from build123d import *

# Parameters (mm, degrees)
SKETCH1_R           = 3
SKETCH1_R_2         = 5
BOSS_EXTRUDE1_DEPTH = 4
FILLET1_R           = 5
SKETCH2_R           = 5
BOSS_EXTRUDE2_DEPTH = 12
SKETCH4_R           = 2.401871641
CUT_EXTRUDE2_DEPTH  = 30
SKETCH6_R           = 2.15
CUT_EXTRUDE3_DEPTH  = 2.9


with BuildPart() as part:
    # Sketch1 → Boss-Extrude1 (new body)
    with BuildSketch(Plane(origin=(0, 0, 0), x_dir=(1, 0, 0), z_dir=(0, 1, 0))):
        Polygon((-5.790326763, 58.347363117), (-5.790326763, -9.85213545), (63.193084095, -9.85213545), align=None)
        with Locations(Location((2.52138652, 36.496379496, 0), (0, 0, 270))):
            Circle(SKETCH1_R, mode=Mode.SUBTRACT)
        with Locations(Location((34.519986489, 4.856379496, 0), (0, 0, 270))):
            Circle(SKETCH1_R_2, mode=Mode.SUBTRACT)
    extrude(amount=BOSS_EXTRUDE1_DEPTH)

    # Fillet1
    fillet1_edges = [part.edges().sort_by_distance(p)[0] for p in [
        (63.193084095, 2, 9.85213545),
        (-5.790326763, 2, -58.347363117),
    ]]
    fillet(fillet1_edges, radius=FILLET1_R)

    # Sketch2 → Boss-Extrude2 (add)
    # profile 1 of 5: a face of its own
    with BuildSketch(Plane(origin=(0, 4, 0), x_dir=(1, 0, 0), z_dir=(0, 1, 0))):
        with BuildLine():
            Line((42.017536623, -1.29645629), (54.539062539, -1.29645629))
            Line((54.539062539, -1.29645629), (41.338915092, 11.753687589))
            ThreePointArc((41.338915092, 11.753687589), (43.470054942, 8.593613888), (44.21898882, 4.856379496))
            ThreePointArc((44.21898882, 4.856379496), (43.65205642, 1.588973033), (42.017536623, -1.29645629))
        make_face()
    # profile 2 of 5: a face of its own
    with BuildSketch(Plane(origin=(0, 4, 0), x_dir=(1, 0, 0), z_dir=(0, 1, 0))):
        with BuildLine():
            ThreePointArc((51.023789334, -9.85213545), (55.648635051, -6.752346517), (54.539062539, -1.29645629))
            Line((54.539062539, -1.29645629), (42.017536623, -1.29645629))
            ThreePointArc((42.017536623, -1.29645629), (34.519986489, -4.842622834), (27.022436356, -1.29645629))
            Line((27.022436356, -1.29645629), (-5.790326763, -1.29645629))
            Line((-5.790326763, -1.29645629), (-5.790326763, -9.85213545))
            Line((-5.790326763, -9.85213545), (51.023789334, -9.85213545))
        make_face()
    # profile 3 of 5: a face of its own
    with BuildSketch(Plane(origin=(0, 4, 0), x_dir=(1, 0, 0), z_dir=(0, 1, 0))):
        with BuildLine():
            ThreePointArc((27.022436356, -1.29645629), (34.519986489, -4.842622834), (42.017536623, -1.29645629))
            Line((42.017536623, -1.29645629), (27.022436356, -1.29645629))
        make_face()
    # profile 4 of 5: a face of its own
    with BuildSketch(Plane(origin=(0, 4, 0), x_dir=(1, 0, 0), z_dir=(0, 1, 0))):
        with BuildLine():
            ThreePointArc((34.519986489, 14.555381827), (38.206016803, 13.827657373), (41.338915092, 11.753687589))
            Line((41.338915092, 11.753687589), (32.887372323, 20.109188887))
            Line((32.887372323, 20.109188887), (-5.790326763, 20.109188887))
            Line((-5.790326763, 20.109188887), (-5.790326763, 14.555381827))
            Line((-5.790326763, 14.555381827), (34.519986489, 14.555381827))
        make_face()
    # profile 5 of 5: a face of its own
    with BuildSketch(Plane(origin=(0, 4, 0), x_dir=(1, 0, 0), z_dir=(0, 1, 0))):
        with BuildLine():
            Line((27.022436356, -1.29645629), (42.017536623, -1.29645629))
            ThreePointArc((42.017536623, -1.29645629), (43.65205642, 1.588973033), (44.21898882, 4.856379496))
            ThreePointArc((44.21898882, 4.856379496), (43.470054942, 8.593613888), (41.338915092, 11.753687589))
            ThreePointArc((41.338915092, 11.753687589), (38.206016803, 13.827657373), (34.519986489, 14.555381827))
            ThreePointArc((34.519986489, 14.555381827), (25.752232648, 9.003322803), (27.022436356, -1.29645629))
        make_face()
        with Locations(Location((34.519986489, 4.856379496, 0), (0, 0, 270))):
            Circle(SKETCH2_R, mode=Mode.SUBTRACT)
    extrude(amount=BOSS_EXTRUDE2_DEPTH)

    # Sketch4 → Cut-Extrude2 (cut)
    with BuildSketch(Plane(origin=(0, 0, 1.29645629), x_dir=(-1, 0, 0), z_dir=(0, 0, -1))):
        with Locations((-14.209673237, 10)):
            Circle(SKETCH4_R)
    extrude(amount=-CUT_EXTRUDE2_DEPTH, mode=Mode.SUBTRACT)

    # Sketch6 → Cut-Extrude3 (cut)
    with BuildSketch(Plane(origin=(0, 16, 0), x_dir=(1, 0, 0), z_dir=(0, 1, 0))):
        with Locations(Location((46.209673237, -5.58213545, 0), (0, 0, 270))):
            Circle(SKETCH6_R)
        with Locations(Location((4.209673237, -5.58213545, 0), (0, 0, 270))):
            Circle(SKETCH6_R)
    extrude(amount=-CUT_EXTRUDE3_DEPTH, mode=Mode.SUBTRACT)


solid = part.part
Geometry: final body of the model. Coordinates: model frame, mm. A direction names the side the tool comes from. Round coordinates to 2 decimals unless told otherwise and drop trailing zeros. Loops run counter-clockwise (first coordinate to the right, second up) from the corner with the lowest first, then second, coordinate; pieces in that order, holes last.
Q1. Material intervals for L1, parallel to Z at x = 17.5, y = 8; L2, parallel to Z at x = 31, y = 4.75; L3, parallel to X at y = 15.75, z = -8.5, sorted ascending.
Q2. Section A-A on y = 10. Return loops of the section in (x, z).
Q3. Section D-D on z = -34.5. Return loops of the section in (x, y), plus the area to 3 significant figures.
Q4. Pull-direction query (X, two-part tool) for faces 1 (the flat face through (46, 13.1, 6)), 2 (the cylindrical face through (14.73, 7.655, 5.514)), 3 (the flat face through (-5.79, 3, -12)), 4 (the cylindrical face through (-2.793, 2.028, -50.955)); classes: released by +X, released by -X, zero draft, split by the parting line, or undercut.
Q5. Pin query (flat end, axial travel): P1, Ø12.5, axis at x = 14, z = -6.5, coming from the +Y side; P2, Ø3.5, axis at x = 4, z = 5.5, coming from the +Y side; P3, Ø6, axis at x = 12.5, y = 9, coming from the -Z side; P4, Ø2, axis at x = 26, z = -30, coming from the +Y side. Return the tip coordinate at first contact, or that it passes through.
Q6. Access query for faces 5 (the flat face through (11, 10, 1.296)), 6 (the cylindrical face through (44.901, 14.57, 3.876)), 7 (the flat face through (9, 4, -32)). Directions: +Z, -Z, +X, -X, +Y, -Y. A direction counts if a zero-diameter tool reaches every point of the face in a straight line with its end or side. Return the directions, or none.
Q7. Section C-C on x = 24. Return loops of the section in (y, z).
Q8. Section B-B on y = 5.25. Return loops of the section in (x, z), plus the area to 3 significant figures.
Evaluation:
1. L1: z = -20.11 to -14.56, 1.3 to 9.85
1. L2: z = -20.11 to -14.56, -13.89 to -8.41, -1.31 to 9.85
1. L3: x = 25.53 to 31.1, 37.94 to 44.63
2. outline: (-5.79, -20.11) - (32.89, -20.11) - (54.54, 1.3) arc R5 ccw to (51.02, 9.85) - (16.61, 9.85) - (16.61, 1.3) - (27.02, 1.3) arc R9.7 ccw to (34.52, -14.56) - (-5.79, -14.56) - close; (-5.79, 1.3) - (11.81, 1.3) - (11.81, 9.85) - (-5.79, 9.85) - close; hole circle Ø10 at (34.52, -4.86)
3. outline: (-5.79, 0) - (0.28, 0) - (0.28, 4) - (-5.79, 4) - close; (4.76, 0) - (18.33, 0) - (18.33, 4) - (4.76, 4) - close
3. area: 78.6 mm2
4. face 1: undercut
4. face 2: undercut
4. face 3: released by -X
4. face 4: split by the parting line
5. P1: stops at y = 4
5. P2: stops at y = 13.1
5. P3: stops at z = -20.11
5. P4: passes through
6. face 5: -X, +Y
6. face 6: +Y
6. face 7: -Z, +X, -X, +Y
7. outline: (0, -28.9) - (4, -28.9) - (4, -20.11) - (16, -20.11) - (16, -14.56) - (4, -14.56) - (4, 1.3) - (16, 1.3) - (16, 9.85) - (0, 9.85) - close
8. outline: (-5.79, -20.11) - (32.89, -20.11) - (54.54, 1.3) arc R5 ccw to (51.02, 9.85) - (-5.79, 9.85) - (-5.79, 1.3) - (27.02, 1.3) arc R9.7 ccw to (34.52, -14.56) - (-5.79, -14.56) - close; hole circle Ø10 at (34.52, -4.86)
8. area: 993 mm2
